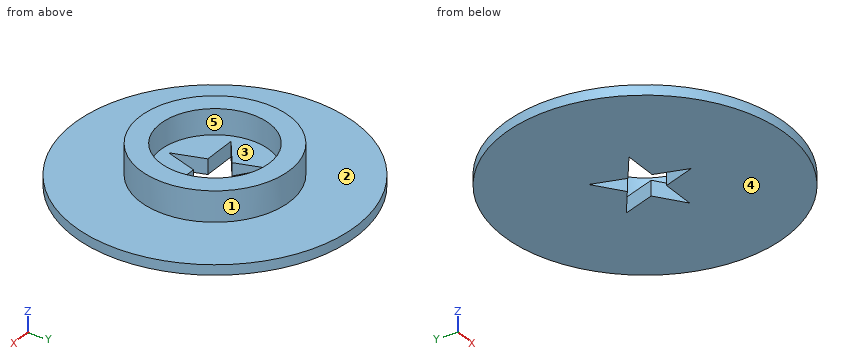
from build123d import *

# Parameters (mm, degrees)
F3_DEPTH = 25


with BuildPart() as f1:
    # F0 (on Front) → F1 (revolve)
    with BuildSketch(Plane.XZ):
        Polygon((0, 1.5), (0, 0), (14, 0), (14, 1), (7.4, 1), (7.4, 4), (5.4, 4), (5.4, 1.5), align=None)
    revolve(axis=Axis((0, 0, 0.75), (0, 0, -1)))

    # F2 (on face) → F3 (cut)
    with BuildSketch(Plane.XY.offset(1.5)):
        Polygon((-1.0285587608, -1.4156896825), (-1.6642430343, 0.5407453412), (-4.3570448294, -1.4156896825), align=None)
        Polygon((0, 1.7498886826), (-2.6928017951, 3.7063237062), (-1.6642430343, 0.5407453412), align=None)
        Polygon((1.6642430343, 0.5407453412), (0, 1.7498886826), (-1.6642430343, 0.5407453412), (-1.0285587608, -1.4156896825), (1.0285587608, -1.4156896825), align=None)
        Polygon((2.6928017951, 3.7063237062), (0, 1.7498886826), (1.6642430343, 0.5407453412), align=None)
        Polygon((4.3570448294, -1.4156896825), (1.6642430343, 0.5407453412), (1.0285587608, -1.4156896825), align=None)
        Polygon((1.0285587608, -1.4156896825), (-1.0285587608, -1.4156896825), (0, -4.5812680475), align=None)
    extrude(amount=-F3_DEPTH, mode=Mode.SUBTRACT)


solid = f1.part
Verification items for the finished model (mm, model axes). Face numbers are marked on the shaded views. A direction names the side the tool comes from. Coordinates: 2 decimals unless noted, no trailing zeros. Loops run counter-clockwise (first coordinate to the right, second up) from the corner with the lowest first, then second, coordinate; pieces in that order, holes last. Notation, with made-up numbers: (56.5, -29.75) -> (102.5, -29.75) arc R8 ccw to (102.5, -21.75) -> close; hole circle Ø2 at (14.25, 61). An arc over 180 degrees is marked (long way). Answer as CSV lines item,"result".
1) Cross-section at A-A, the plane x = -2. Record the cut outline in (y, z).
Found:
outline,"(-13.86, 0) -> (-1.42, 0) -> (-1.42, 1.5) -> (-5.02, 1.5) -> (-5.02, 4) -> (-7.12, 4) -> (-7.12, 1) -> (-13.86, 1) -> close; (0.3, 0) -> (1.57, 0) -> (1.57, 1.5) -> (0.3, 1.5) -> close; (3.2, 0) -> (13.86, 0) -> (13.86, 1) -> (7.12, 1) -> (7.12, 4) -> (5.02, 4) -> (5.02, 1.5) -> (3.2, 1.5) -> close"
2) Cross-section at B-B, the plane y = 0. Record the cut outline in (x, z), then the cut area to 3 significant figures.
Found:
outline,"(-14, 0) -> (-2.41, 0) -> (-2.41, 1.5) -> (-5.4, 1.5) -> (-5.4, 4) -> (-7.4, 4) -> (-7.4, 1) -> (-14, 1) -> close; (2.41, 0) -> (14, 0) -> (14, 1) -> (7.4, 1) -> (7.4, 4) -> (5.4, 4) -> (5.4, 1.5) -> (2.41, 1.5) -> close"
area,"38.2 mm2"
3) Cross-section at C-C, the plane y = -6. Record the cut outline in (x, z), then the cut area to 3 significant figures.
Found:
outline,"(-12.65, 0) -> (12.65, 0) -> (12.65, 1) -> (4.33, 1) -> (4.33, 4) -> (-4.33, 4) -> (-4.33, 1) -> (-12.65, 1) -> close"
area,"51.3 mm2"
4) Cross-section at D-D, the plane x = -10.5. Record the cut outline in (y, z).
Found:
outline,"(-9.26, 0) -> (9.26, 0) -> (9.26, 1) -> (-9.26, 1) -> close"
5) Tool access check on the marked faces 4 and 5. Record the directions out of +Z, -Z, +X, -X, +Y, -Y that give a thin tool (end or side, any length) a straight path to the whole face; none if there is none.
Found:
face 4,"-Z, +X, -X, +Y, -Y"
face 5,"+Z"
6) Release check for a two-part mould opening along Y. For the marked faces 1, 2 and 3 record: +Y half, -Y half, draft (parallel to the pull), parting line (faces both ways), or undercut.
Found:
face 1,"parting line"
face 2,"draft"
face 3,"undercut"
7) Depth check by flat-ended pin: pin 1 (0.8 mm diameter, centred on x = -3, z = 1, fed in from +Y); pin 2 (1 mm diameter, centred on x = 6, z = 2, fed in from +Y); pin 3 (1 mm diameter, centred on y = -4, z = 3, fed in from +X). Enter the tip coordinate at first touch or a pass-through.
Found:
pin 1,"stops at y = 13.76"
pin 2,"stops at y = 4.95"
pin 3,"stops at x = 6.52"
8) Thickness scan on L1, parallel to X at y = 0, z = 3.4; L2, parallel to Z at x = -6.5, y = -6.5. Record the ranges inside material, lowest first. Write a range as from..to.
Found:
L1,"x = -7.4..-5.4, 5.4..7.4"
L2,"z = 0..1"
